Verification items for the finished model (mm, model axes). A direction names the side the tool comes from. Give positions to 0.01 mm unless a question says otherwise; leave off trailing zeros. Write each loop counter-clockwise with the first axis right and the second up, starting at its lowest first coordinate (ties: lowest second). Pieces come first, ordered by that corner, then holes. Notation, with made-up numbers: (89, -33) -> (123, -33) arc R17 cw to (123, -7) -> close; hole circle Ø5 at (89, 74). An arc over 180 degrees is marked (long way). Write item = value, one per line.
Autodesk Inventor part; units mm, degrees
ref_plane "YZ Plane" through (0, 0, 0) normal (1, 0, 0) x (0, 1, 0)
ref_plane "XZ Plane" through (0, 0, 0) normal (0, 1, 0) x (-1, 0, 0)
ref_plane "XY Plane" through (0, 0, 0) normal (0, 0, 1) x (1, 0, 0)
sketch "Sketch1" plane through (0, 0, 0) normal (0, 0, 1) x (1, 0, 0)
  line L0 (0, 0) -> (0, 87.5)
  circle A0 centre (68.0717, 68.3624) radius 50 construction
  line L1 (0, 87.5) -> (43.6046, 111.967)
  line L2 (0, 0) -> (50, 0)
  line L3 (50, 0) -> (93.217, 25.1454)
  arc A1 (93.217, 25.1454) -> (43.6046, 111.967) centre (68.0717, 68.3624) ccw
  dimension "d0" = 87.5
  dimension "d1" = 100
  dimension "d2" = 50
  dimension "d3" = 50
  dimension "d4" = 50
extrude "Extrusion1" add sketch "Sketch1" along normal blind 50
sketch "Sketch3" plane through (0, 0, 0) normal (0, 0, -1) x (-1, 0, 0)
  line L0 (0, 87.5) -> (-43.6046, 111.967)
  arc A0 (-43.6046, 111.967) -> (-93.217, 25.1454) centre (-68.0717, 68.3624) ccw
  line L1 (-93.217, 25.1454) -> (-50, 0)
  line L2 (-50, 0) -> (0, 0)
  line L3 (0, 5) -> (-48.6512, 5)
  line L4 (-48.6512, 5) -> (-90.7025, 29.4671)
  arc A1 (-46.0513, 107.6066) -> (-90.7025, 29.4671) centre (-68.0717, 68.3624) ccw
  line L5 (-46.0513, 107.6066) -> (0, 81.7667)
  line L6 (0, 0) -> (0, 87.5)
  line L7 (0, 5) -> (0, 81.7667)
  line L8 (0, 87.5) -> (0, 0)
  dimension "d10" = 5
extrude "Extrusion3" cut sketch "Sketch3" against normal blind 45 contours L6 L3 L4 A1 L5
sketch "Sketch4" plane through (0, 0, 45) normal (0, 0, -1) x (-1, 0, 0)
  arc A0 (-43.6046, 111.967) -> (-93.217, 25.1454) centre (-68.0717, 68.3624) ccw
  circle A1 centre (-68.0717, 68.3624) radius 6.25
  point P0 (0, 0)
  dimension "d13" = 12.5
extrude "Extrusion4" cut sketch "Sketch4" against normal through all
sketch "Sketch5" plane through (0, 0, 45) normal (0, 0, -1) x (-1, 0, 0)
  circle A0 centre (-68.0717, 68.3624) radius 6.25
  circle A1 centre (-68.0717, 68.3624) radius 6.25
  circle A2 centre (-68.0717, 68.3624) radius 21.25
  point P0 (0, 0)
  dimension "d16" = 15
extrude "Extrusion5" add sketch "Sketch5" along normal blind 35
sketch "Sketch6" plane through (0, 0, 50) normal (0, 0, 1) x (1, 0, 0)
  circle A0 centre (68.0717, 68.3624) radius 21.25
  point P0 (0, 0)
extrude "Extrusion6" add sketch "Sketch6" along normal blind 5
sketch "Sketch7" plane through (0, 0, 0) normal (0, 0, -1) x (-1, 0, 0)
  arc A0 (-43.6046, 111.967) -> (-93.217, 25.1454) centre (-68.0717, 68.3624) ccw
  line L0 (-18.0717, 68.3624) -> (-18.0717, 97.6402)
  line L1 (0, 87.5) -> (-43.6046, 111.967)
  line L2 (-18.0717, 97.6402) -> (-43.6046, 111.967)
  line L3 (-68.0717, 18.3624) -> (-81.5592, 18.3624)
  line L4 (-93.217, 25.1454) -> (-50, 0)
  line L5 (-50, 0) -> (-93.217, 25.1454)
  line L6 (-81.5592, 18.3624) -> (-93.217, 25.1454)
  arc A1 (-93.217, 25.1454) -> (-68.0717, 18.3624) centre (-68.0717, 68.3624) ccw
  arc A2 (-43.6046, 111.967) -> (-93.217, 25.1454) centre (-68.0717, 68.3624) ccw
  arc A3 (-18.0717, 68.3624) -> (-43.6046, 111.967) centre (-68.0717, 68.3624) ccw
  circle A4 centre (-68.0717, 68.3624) radius 50
  point P0 (0, 0)
extrude "Extrusion7" cut sketch "Sketch7" against normal blind 10
sketch "Sketch8" plane through (0, 0, 45) normal (0, 0, -1) x (-1, 0, 0)
  circle A0 centre (-21.5, 30) radius 5
  circle A1 centre (-21.5, 30) radius 15
  line L0 (-50, 0) -> (0, 0)
  line L1 (0, 0) -> (0, 5)
  dimension "d23" = 10
  dimension "d24" = 30
  dimension "d25" = 30
  dimension "d26" = 21.5
extrude "Extrusion8" add sketch "Sketch8" along normal blind 45
sketch "Sketch9" plane through (0, 0, 50) normal (-1, 0, 0) x (0, 0, 1)
  line L0 (0, 87.5) -> (-50, 87.5)
  line L1 (-50, 87.5) -> (-50, 72.5)
  line L2 (-50, 72.5) -> (0, 72.5)
  line L3 (0, 72.5) -> (0, 87.5)
  line L4 (0, 87.5) -> (-15, 87.5)
  line L5 (-15, 87.5) -> (-15, 32.5)
  line L6 (-15, 32.5) -> (0, 32.5)
  line L7 (0, 32.5) -> (0, 87.5)
  line L8 (-50, 0) -> (0, 0)
  dimension "d29" = 50
  dimension "d30" = 15
  dimension "d31" = 15
  dimension "d32" = 32.5
extrude "Extrusion9" add sketch "Sketch9" against normal blind 5
sketch "Sketch10" plane through (0, 0, 45) normal (0, 0, -1) x (-1, 0, 0)
  circle A0 centre (-15, 78.7167) radius 10
  circle A1 centre (-15, 78.7167) radius 6
  line L0 (-18.0717, 91.9069) -> (-5, 84.5722)
  line L1 (-5, 72.5) -> (-5, 84.5722)
  point P0 (0, 0)
  dimension "d35" = 20
  dimension "d36" = 12
extrude "Extrusion10" add sketch "Sketch10" along normal blind 45 contours A0
sketch "Sketch11" plane through (0, 0, 0) normal (0, 0, -1) x (-1, 0, 0)
  circle A0 centre (-15, 78.7167) radius 6
  circle A1 centre (-15, 78.7167) radius 2.5
  point P0 (0, 0)
  dimension "d39" = 5
extrude "Extrusion11" add sketch "Sketch11" against normal blind 10
sketch "Sketch13" plane through (0, 0, 50) normal (0, 0, 1) x (1, 0, 0)
  circle A0 centre (15, 78.7167) radius 6
  point P0 (0, 0)
extrude "Extrusion12" cut sketch "Sketch13" against normal blind 5
sketch "Sketch14" plane through (68.0717, 68.3624, 55) normal (0, 0, 1) x (1, 0, 0)
  circle A0 centre (0, 0) radius 2.5
  circle A1 centre (0, 0) radius 21.25
  circle A2 centre (-46.5717, -38.3624) radius 15
  circle A3 centre (-46.5717, -38.3624) radius 2.5
  point P0 (-68.0717, -68.3624)
  dimension "d44" = 5
  dimension "d47" = 5
extrude "Extrusion13" cut sketch "Sketch14" against normal through all contours A0 | A3
properties part number "BA004" material "ABS Plastic"
Item 1: Set-up check for faces 1 (the flat face through (45, 60, 50)), 2 (the flat face through (77, 18.362, 5)), 3 (the flat face through (2, 32.5, 40)): record each of +Z, -Z, +X, -X, +Y, -Y from which the full face is reachable in a straight line by a thin tool's end or side.
Response values:
face_1 = +Z
face_2 = -Z, +X, +Y
face_3 = -Z, -X
Item 2: Material ranges on line 1 (Y direction, x = 53, z = 43); line 2 (X direction, y = 36.5, z = 39.5); line 3 (X direction, y = 27, z = 19), recorded low to high.
Response values:
line_1 = 1.75 to 7.53, 53.38 to 83.34, 110.76 to 116.04
line_2 = 0 to 5, 7.98 to 35.02, 99.85 to 106.6
line_3 = 6.8 to 17.5, 25.5 to 36.2, 86.46 to 96.16
Item 3: Go/stop test with flat-tipped pins: P1, Ø3, axis at x = 68.07, y = 68.36, coming from the +Z side; P2, Ø3, axis at x = 43.5, y = 47, coming from the +Z side; P3, Ø13, axis at x = 70.5, y = 76, coming from the -Z side; P4, Ø11, axis at x = 68.07, y = 68.36, coming from the -Z side. Record where each tip stops, or that it passes through.
Response values:
P1 = through
P2 = 50
P3 = 10
P4 = 50
Item 4: Mould release check, pull along Y, two halves, no side actions. Record for faces 4 (the flat face through (2, 72.5, 17)), 5 (the cylindrical face through (111, 94, 30)), 6 (the flat face through (24, 5, 22)), 7 (the flat face through (41, 4, 0)): +Y half, -Y half, draft (parallel to the pull), parting line (faces both ways), or undercut.
Response values:
face_4 = undercut
face_5 = parting line
face_6 = undercut
face_7 = draft
Item 5: Sectioned sample at D-D on x = 80. Record the cut outline in (y, z), then the cut area to 3 significant figures.
Response values:
outline = (17.46, 0) -> (18.36, 0) -> (18.36, 10) -> (23.24, 10) -> (23.24, 45) -> (50.78, 45) -> (50.78, 10) -> (85.95, 10) -> (85.95, 45) -> (111.75, 45) -> (111.75, 10) -> (116.92, 10) -> (116.92, 50) -> (85.95, 50) -> (85.95, 55) -> (50.78, 55) -> (50.78, 50) -> (17.46, 50) -> close
area = 2,300 mm^2
Item 6: Sectioned sample at C-C on x = 15. Record the cut outline in (y, z).
Response values:
outline = (0, 0) -> (5, 0) -> (5, 45) -> (16.48, 45) -> (16.48, 0) -> (43.52, 0) -> (43.52, 45) -> (68.72, 45) -> (68.72, 0) -> (76.22, 0) -> (76.22, 10) -> (72.72, 10) -> (72.72, 50) -> (0, 50) -> close; (81.22, 0) -> (88.72, 0) -> (88.72, 45) -> (90.18, 45) -> (90.18, 0) -> (95.92, 0) -> (95.92, 50) -> (84.72, 50) -> (84.72, 10) -> (81.22, 10) -> close
